Geometry check sheet. Reference: the model listing, model coordinates, mm. Face numbers are marked on the shaded views. A direction names the side the tool comes from. Round coordinates to 2 decimals unless told otherwise and drop trailing zeros. Loops run counter-clockwise (first coordinate to the right, second up) from the corner with the lowest first, then second, coordinate; pieces in that order, holes last. Notation, with made-up numbers: M 36.5,84 L 75.5,84 A19 ccw 75.5,96 Z; hole C 2,-9.5 d4. An arc over 180 degrees is marked long. Answer in a Markdown table with one row per item. Add a question column.
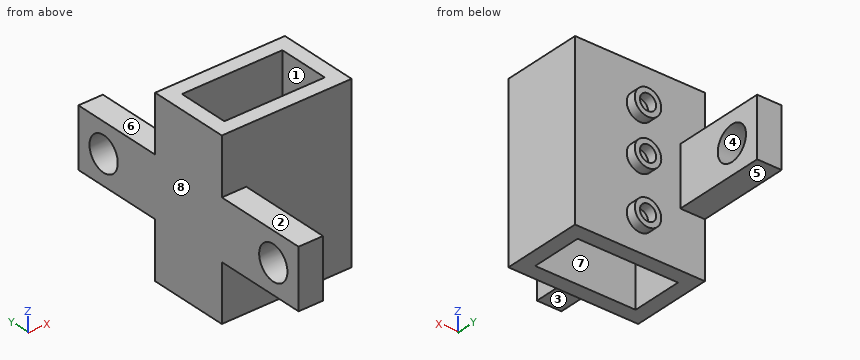
```python
from build123d import *

# Parameters (mm, degrees)
F0_W      = 26.5
F0_H      = 35
F1_DEPTH  = 16.5
F2_W      = 20.5
F2_H      = 10.5
F3_DEPTH  = 35
F4_R      = 2.7
F4_R_2    = 1.65
F5_DEPTH  = 2
F6_W      = 5
F6_H      = 12
F7_DEPTH  = 19
F8_W      = 5
F8_H      = 12
F9_DEPTH  = 19
F10_R     = 3.5
F11_DEPTH = 5
F12_R     = 3.5
F13_DEPTH = 5


with BuildPart() as f1:
    # F0 (on Front) → F1 (new body)
    with BuildSketch(Plane.XZ):
        Rectangle(F0_W, F0_H)
    extrude(amount=F1_DEPTH)

    # F2 (on face) → F3 (cut)
    with BuildSketch(Plane.XY.offset(17.5)):
        with Locations((0, -8.25)):
            Rectangle(F2_W, F2_H)
    extrude(amount=-F3_DEPTH, mode=Mode.SUBTRACT)

    # F4 (on face) → F5 (join)
    with BuildSketch(Plane(origin=(0, 0, 0), x_dir=(-1, 0, 0), z_dir=(0, 1, 0))):
        Circle(F4_R)
        Circle(F4_R_2, mode=Mode.SUBTRACT)
        with Locations((0, 9.5)):
            Circle(F4_R)
        with Locations((0, 9.5)):
            Circle(F4_R_2, mode=Mode.SUBTRACT)
        with Locations((0, -11)):
            Circle(F4_R)
        with Locations((0, -11)):
            Circle(F4_R_2, mode=Mode.SUBTRACT)
    extrude(amount=F5_DEPTH)

    # F6 (on face) → F7 (join)
    with BuildSketch(Plane.XZ.offset(16.5)):
        with Locations((-10.75, 0)):
            Rectangle(F6_W, F6_H)
    extrude(amount=F7_DEPTH)

    # F8 (on face) → F9 (join)
    with BuildSketch(Plane(origin=(0, 0, 0), x_dir=(-1, 0, 0), z_dir=(0, 1, 0))):
        with Locations((10.75, 0)):
            Rectangle(F8_W, F8_H)
    extrude(amount=F9_DEPTH)

    # F10 (on face) → F11 (cut)
    with BuildSketch(Plane.YZ.offset(-8.25)):
        with Locations((12.75, 0)):
            Circle(F10_R)
    extrude(amount=-F11_DEPTH, mode=Mode.SUBTRACT)

    # F12 (on face) → F13 (cut)
    with BuildSketch(Plane.YZ.offset(-8.25)):
        with Locations((-29.25, 0)):
            Circle(F12_R)
    extrude(amount=-F13_DEPTH, mode=Mode.SUBTRACT)


solid = f1.part
```
1) Go/stop test with flat-tipped pins: pin 1 (3.5 mm diameter, centred on y = -27.5, z = 2, fed in from +X); pin 2 (1 mm diameter, centred on x = 9, y = -9.5, fed in from +Z); pin 3 (5.5 mm diameter, centred on x = -11, y = -22, fed in from +Z); pin 4 (4 mm diameter, centred on x = 0, z = 9.5, fed in from -Y). Record where each tip stops, or that it passes through.
2) Cross-section at A-A, the plane x = 6.75. Record the boundary of the cut face in (y, z), plus the area to 3 significant figures.
3) Cross-section at D-D, the plane z = 9.5. Record the boundary of the cut face in (x, y).
4) Cross-section at C-C, the plane y = 12.75. Record the boundary of the cut face in (x, z).
5) Draft check along X on the marked faces 6, 7 and 8. Enter one of: +X half, -X half, draft (parallel to the pull), parting line (faces both ways), or undercut.
6) Set-up check for the marked faces 1, 2, 3, 4 and 5: record each of +Z, -Z, +X, -X, +Y, -Y from which the full face is reachable in a straight line by a thin tool's end or side.
7) Cross-section at B-B, the plane z = 0. Record the boundary of the cut face in (x, y).
8) Thickness scan on L1, parallel to Y at x = -2.5, z = 15; L2, parallel to X at y = -10, z = 9; L3, parallel to Z at x = -10.75, y = -17. Record the ranges inside material, lowest first. Write a range as [from, to].
Worked answers:
| question | item | result |
|---|---|---|
| 1 | pin 1 | stops at x = -8.25 |
| 1 | pin 2 | passes through |
| 1 | pin 3 | stops at z = 6 |
| 1 | pin 4 | stops at y = -16.5 |
| 2 | outline | M -16.5,-17.5 L -13.5,-17.5 L -13.5,17.5 L -16.5,17.5 Z; M -3,-17.5 L 0,-17.5 L 0,17.5 L -3,17.5 Z |
| 2 | area | 210 mm2 |
| 3 | outline | M -13.25,-16.5 L 13.25,-16.5 L 13.25,0 L 2.7,0 L 2.7,2 L 1.65,2 L 1.65,0 L -1.65,0 L -1.65,2 L -2.7,2 L -2.7,0 L -13.25,0 Z; hole M -10.25,-13.5 L 10.25,-13.5 L 10.25,-3 L -10.25,-3 Z |
| 4 | outline | M -13.25,-6 L -8.25,-6 L -8.25,-3.5 L -13.25,-3.5 Z; M -13.25,3.5 L -8.25,3.5 L -8.25,6 L -13.25,6 Z |
| 5 | face 6 | draft |
| 5 | face 7 | undercut |
| 5 | face 8 | -X half |
| 6 | face 1 | +Z, -Z |
| 6 | face 2 | +Z, +X, -X, -Y |
| 6 | face 3 | -Z, +X, -X, -Y |
| 6 | face 4 | +X, -X |
| 6 | face 5 | -Z, +X, -X, +Y |
| 7 | outline | M -13.25,-35.5 L -8.25,-35.5 L -8.25,-32.75 L -13.25,-32.75 Z; M -13.25,-25.75 L -8.25,-25.75 L -8.25,-16.5 L 13.25,-16.5 L 13.25,0 L 2.7,0 L 2.7,2 L 1.65,2 L 1.65,0 L -1.65,0 L -1.65,2 L -2.7,2 L -2.7,0 L -8.25,0 L -8.25,9.25 L -13.25,9.25 Z; M -13.25,16.25 L -8.25,16.25 L -8.25,19 L -13.25,19 Z; hole M -10.25,-13.5 L 10.25,-13.5 L 10.25,-3 L -10.25,-3 Z |
| 8 | L1 | y = [-16.5, -13.5], [-3, 0] |
| 8 | L2 | x = [-13.25, -10.25], [10.25, 13.25] |
| 8 | L3 | z = [-6, 6] |
